Can you work these out from the model? Positions are in its coordinate system, mm. Give positions to 0.01 mm unless a question says otherwise; leave off trailing zeros. Write each loop counter-clockwise with the first axis right and the second up, starting at its lowest first coordinate (ties: lowest second). Pieces come first, ordered by that corner, then holes. Notation, with made-up numbers: M 1,13 L 20,13 A24 ccw 20,44 Z; hole C -26,4.5 d2. An arc over 180 degrees is marked long. Use CSV: the item, a comma, the result in double quotes. Start each with the question number.
from build123d import *

# Parameters (mm, degrees)
BOSS_EXTRUDE1_DEPTH        = 19.05
BOSS_EXTRUDE2_DEPTH        = 19.05
FILLET1_R                  = 3.175
FILLET2_R                  = 12.7
CUT_EXTRUDE1_DEPTH         = 965.552600368
CUT_EXTRUDE1_DEPTH_BACK    = 965.552600368
SKETCH47_R                 = 3.175
FILLET4_R                  = 6.35
F_1_2_0_5_DIAMETER_HOLE1_D = 12.7
HOLE7_D                    = 3.175
HOLE7_DEPTH                = 38.1
HOLE7_CSINK_D              = 10.16
HOLE7_CSINK_ANGLE          = 82
HOLE7_TIP                  = 0.953866233
HOLE10_D                   = 3.175
HOLE10_DEPTH               = 57.15
HOLE10_CSINK_D             = 10.16
HOLE10_CSINK_ANGLE         = 82
HOLE10_TIP                 = 0.953866233
HOLE13_D                   = 3.175
HOLE13_DEPTH               = 31.75
HOLE13_CSINK_D             = 10.16
HOLE13_CSINK_ANGLE         = 82
HOLE13_TIP                 = 0.953866233


with BuildPart() as part:
    # Sketch1 → Boss-Extrude1 (new body)
    with BuildSketch(Plane.XY):
        Polygon((-247.274665566, 82.142339986), (-327.22102196, 55.917162383), (-560.337153612, 766.561933763), (-504.525442447, 784.870110692), (-417.251419261, 518.818903446), (-393.116774032, 526.735904121), align=None)
    extrude(amount=-BOSS_EXTRUDE1_DEPTH)

    # Sketch2 → Boss-Extrude2 (add, through all)
    with BuildSketch(Plane.XY):
        Polygon((-393.116774032, 526.735904121), (-336.901176267, 355.36500697), (-277.604402796, 374.816405204), (-281.415155825, 417.005352091), (-320.44916939, 493.083731154), (-290.280862854, 502.979981998), (-307.307307279, 554.884385267), align=None)
    extrude(amount=-BOSS_EXTRUDE2_DEPTH)

    # Fillet1
    fillet1_edges = [part.edges().sort_by_distance(p)[0] for p in [
        (-320.44916939, 493.083731154, -9.525),
    ]]
    fillet(fillet1_edges, radius=FILLET1_R)

    # Fillet2
    fillet2_edges = [part.edges().sort_by_distance(p)[0] for p in [
        (-336.901176267, 355.36500697, -9.525),
    ]]
    fillet(fillet2_edges, radius=FILLET2_R)

    # Sketch47 → Cut-Extrude1 (cut, two sides: drawn at the far end of the back side and taken through both)
    with BuildSketch(Plane(origin=(0, 0, -19.05), x_dir=(-1, 0, 0), z_dir=(0, 0, -1)).offset(-CUT_EXTRUDE1_DEPTH_BACK)):
        with Locations((417.251419261, 518.818903446)):
            Circle(SKETCH47_R)
    extrude(amount=CUT_EXTRUDE1_DEPTH + CUT_EXTRUDE1_DEPTH_BACK, mode=Mode.SUBTRACT)

    # Fillet4
    fillet4_edges = [part.edges().sort_by_distance(p)[0] for p in [
        (-418.241044345, 521.8357341, -9.525),
        (-414.234588607, 519.80852853, -9.525),
    ]]
    fillet(fillet4_edges, radius=FILLET4_R)

    # 1/2 (0.5) Diameter Hole1 (through all)
    with Locations(Plane.XY):
        with Locations((-563.45033927, 698.544682362), (-504.072834209, 517.534843147), (-316.771364786, 371.99266929), (-323.698740376, 393.110483865), (-289.824308357, 404.222472403), (-287.772364418, 381.505347156), (-305.715281117, 417.978415836), (-364.985283482, 398.535799453), (-384.427899865, 457.805801818), (-325.157897499, 477.248418201), (-332.468536604, 499.165347862), (-305.317060721, 508.071973621), (-316.40575464, 541.875392969), (-343.557230523, 532.968767209)):
            Hole(F_1_2_0_5_DIAMETER_HOLE1_D / 2)

    # Hole7
    with Locations(Plane(origin=(313.774034822, -375.700785937, 19.05), x_dir=(0.9977564584489053, -0.06694811142592419, 0), z_dir=(0, 0, 1))):
        with Locations((-710.914924699, 391.126528253), (-615.24080496, 429.781381762), (-711.83598555, 767.659094962), (-835.937309391, 717.51890547), (-904.68821492, 1078.38439498), (-976.811864753, 1049.244548945)):
            CounterSinkHole(HOLE7_D / 2, HOLE7_CSINK_D / 2, depth=HOLE7_DEPTH, counter_sink_angle=HOLE7_CSINK_ANGLE)
            with Locations((0, 0, -(HOLE7_DEPTH + HOLE7_TIP / 2))):  # 118° drill point
                Cone(0, HOLE7_D / 2, HOLE7_TIP, mode=Mode.SUBTRACT)

    # Hole10
    with Locations(Plane(origin=(313.774034822, -375.700785937, -57.15), x_dir=(-0.9977564584489053, 0.06694811142592419, 0), z_dir=(0, 0, -1))):
        with Locations((848.944412528, 940.413642522), (885.927448463, 1031.949868564), (867.435930496, 986.181755543), (830.452894561, 894.645529501)):
            CounterSinkHole(HOLE10_D / 2, HOLE10_CSINK_D / 2, depth=HOLE10_DEPTH, counter_sink_angle=HOLE10_CSINK_ANGLE)
            with Locations((0, 0, -(HOLE10_DEPTH + HOLE10_TIP / 2))):  # 118° drill point
                Cone(0, HOLE10_D / 2, HOLE10_TIP, mode=Mode.SUBTRACT)

    # Hole13
    with Locations(Plane(origin=(-45.102820315, -493.424841018, 52.974999997), x_dir=(0, 0, -1), z_dir=(0.9501828830204607, 0.3116929399504029, 1.2476428765784286e-15))):
        with Locations((174.999999994, 685.961004241), (174.999999994, 549.837259632), (174.999999994, 413.713515022), (81.549999997, 779.649723129), (81.549999997, 652.344645962), (62.499999997, 662.953402392), (62.499999997, 769.040966698), (-62.499999997, 769.040966698), (-62.499999997, 662.953402392), (-81.549999997, 652.344645962), (-81.549999997, 779.649723129), (-174.999999994, 413.713515022), (-174.999999994, 549.837259632), (-174.999999994, 685.961004241), (-82.737499997, 600.384620239), (0, 600.384620239), (82.737499997, 600.384620239), (0, 376.737770337), (-82.737499997, 376.737770337), (82.737499997, 376.737770337)):
            CounterSinkHole(HOLE13_D / 2, HOLE13_CSINK_D / 2, depth=HOLE13_DEPTH, counter_sink_angle=HOLE13_CSINK_ANGLE)
            with Locations((0, 0, -(HOLE13_DEPTH + HOLE13_TIP / 2))):  # 118° drill point
                Cone(0, HOLE13_D / 2, HOLE13_TIP, mode=Mode.SUBTRACT)


solid = part.part
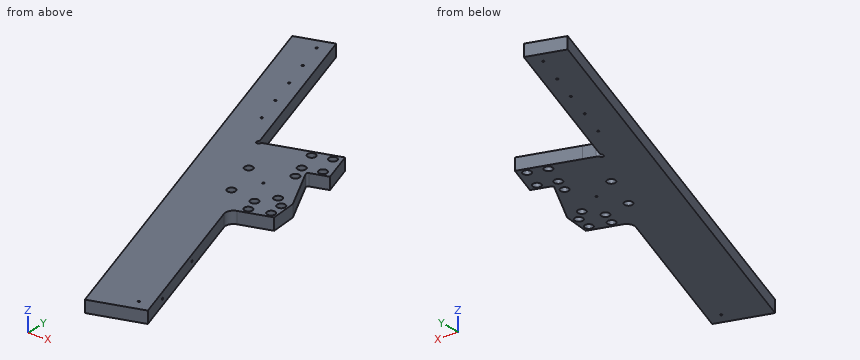
(1) I want a section at C-C (y = 211). Write out the boundary of the cut face in (x, z), and give its area (3 significant figures).
(2) Please list where these lines run through material, in increasing order: L1, parallel to X at y = 516, z = -14; L2, parallel to X at y = 298, z = -18; L3, parallel to X at y = 160.5, z = -17. Write a range as [from, to].
(3) I want a section at A-A (x = -427.5). Write out the boundary of the cut face in (y, z), and give its area (3 significant figures).
(4) Will these pins go through, and if not, where does the flat tip stop? pin 1 Ø7.5 at (x, y) = (-325.16, 477.25) entering from +Z; pin 2 Ø3 at (y, z) = (698, -8) entering from +X; pin 3 Ø5 at (y, z) = (496, -9.5) entering from -X; pin 4 Ø4 at (y, z) = (429, -15) entering from +X.
(5) I want a section at B-B (z = -5). State how many separate pieces and enclosed holes the cut face has, and give its area (3 significant figures).
Geometry results:
1,outline,"M -378.09,-19.05 L -289.54,-19.05 L -289.54,0 L -378.09,0 Z"
1,area,"1,690 mm2"
2,L1,"x = [-478.14, -418.71], [-415.79, -294.55]"
2,L2,"x = [-406.63, -318.08]"
2,L3,"x = [-361.53, -272.98]"
3,outline,"M 361.61,-19.05 L 550.06,-19.05 L 550.06,0 L 361.61,0 Z"
3,area,"3,590 mm2"
4,pin 1,"passes through"
4,pin 2,"stops at x = -475.54"
4,pin 3,"stops at x = -472.4"
4,pin 4,"stops at x = -286.54"
5,separate pieces,"1"
5,enclosed holes,"19"
5,area,"67,500 mm2"
